```python
from build123d import *

# Parameters (mm, degrees)
SKETCH_1_R      = 35
SKETCH_1_R_2    = 15
SKETCH_1_R_3    = 1.6
EXTRUDE_1_DEPTH = 2
SKETCH_2_R      = 24
SKETCH_2_R_2    = 18.6
EXTRUDE_2_DEPTH = 7


with BuildPart() as part:
    # 草图1 → 凸台-拉伸1 (new body)
    with BuildSketch(Plane(origin=(0, 0, 0), x_dir=(1, 0, 0), z_dir=(0, 1, 0))):
        with Locations(Location((0, 0, 0), (0, 0, 270))):
            Circle(SKETCH_1_R)
        with Locations(Location((0, 0, 0), (0, 0, 270))):
            Circle(SKETCH_1_R_2, mode=Mode.SUBTRACT)
        with Locations(Location((29, 0, 0), (0, 0, 270))):
            Circle(SKETCH_1_R_3, mode=Mode.SUBTRACT)
        with Locations(Location((20.506096654, -20.506096654, 0), (0, 0, 270))):
            Circle(SKETCH_1_R_3, mode=Mode.SUBTRACT)
        with Locations(Location((0, -29, 0), (0, 0, 270))):
            Circle(SKETCH_1_R_3, mode=Mode.SUBTRACT)
        with Locations(Location((-20.506096654, -20.506096654, 0), (0, 0, 270))):
            Circle(SKETCH_1_R_3, mode=Mode.SUBTRACT)
        with Locations(Location((-29, 0, 0), (0, 0, 270))):
            Circle(SKETCH_1_R_3, mode=Mode.SUBTRACT)
        with Locations(Location((-20.506096654, 20.506096654, 0), (0, 0, 270))):
            Circle(SKETCH_1_R_3, mode=Mode.SUBTRACT)
        with Locations(Location((0, 29, 0), (0, 0, 270))):
            Circle(SKETCH_1_R_3, mode=Mode.SUBTRACT)
        with Locations(Location((20.506096654, 20.506096654, 0), (0, 0, 270))):
            Circle(SKETCH_1_R_3, mode=Mode.SUBTRACT)
    extrude(amount=-EXTRUDE_1_DEPTH)

    # 草图2 → 凸台-拉伸2 (add)
    with BuildSketch(Plane(origin=(0, 0, 0), x_dir=(1, 0, 0), z_dir=(0, 1, 0))):
        with Locations(Location((0, 0, 0), (0, 0, 270))):
            Circle(SKETCH_2_R)
        with Locations(Location((0, 0, 0), (0, 0, 270))):
            Circle(SKETCH_2_R_2, mode=Mode.SUBTRACT)
    extrude(amount=EXTRUDE_2_DEPTH)


solid = part.part
```
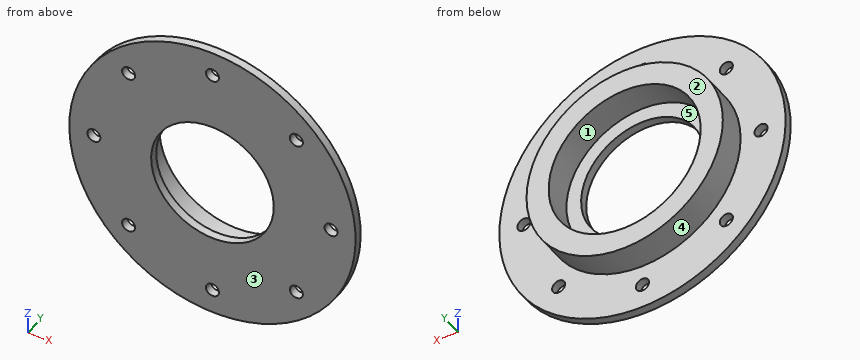
Work out the finished part from the listing and answer in its coordinate system (mm). Face numbers are marked on the shaded views. A direction names the side the tool comes from. Give positions to 0.01 mm unless a question says otherwise; leave off trailing zeros. Order: outer loops, then holes, each group sorted by start corner. A loop starts at its lowest first (then second) coordinate and runs counter-clockwise, first axis right, second up. Notation, with made-up numbers: (-6.75, 51.25) - (31.25, 51.25) arc R32 ccw to (31.25, 83.25) - close; hole circle Ø10 at (29, -5.5). An arc over 180 degrees is marked (long way). One line per item, written item: value. Start each with the question number.
1. Section B-B, the plane z = 29 is taken. Write down the section's boundary in (x, y), then the cut area to 3 significant figures.
2. Section A-A, the plane x = 0 is taken. Write down the section's boundary in (y, z), then the cut area to 3 significant figures.
3. For a pull along Z with two mould halves and no side action, classify the marked faces 3, 4 and 5 as released by +Z, released by -Z, zero draft, split by the parting line, or undercut.
4. Section C-C, the plane x = 10 is taken. Write down the section's boundary in (y, z).
5. Each of these flat-tipped pins is pushed along its axis until it touches: pin 1 Ø3 at (y, z) = (3.5, -4) entering from +X; pin 2 Ø5 at (x, z) = (-20.51, -20.51) entering from +Y. Where does it stop, or does it pass through?
6. Which of the six approach directions +Z, -Z, +X, -X, +Y, -Y give full straight-line access (tool end or side, diameter ignored) to the marked faces 1 and 2?
7. Section D-D, the plane z = -6 is taken. Write down the section's boundary in (x, y), then the cut area to 3 significant figures.
8. Consider line 1 (Y direction, x = 15, z = 3); line 2 (Z direction, x = 13, y = 0.25); line 3 (Z direction, x = 16.5, y = 4). Determine where each line is inside the solid, lowest interval first.
Filled sheet:
1. outline: (-19.6, -2) - (-1.6, -2) - (-1.6, 0) - (-19.6, 0) - close; (1.6, -2) - (19.6, -2) - (19.6, 0) - (1.6, 0) - close
1. area: 72.0 mm²
2. outline: (-2, -35) - (0, -35) - (0, -30.6) - (-2, -30.6) - close; (-2, -27.4) - (0, -27.4) - (0, -24) - (7, -24) - (7, -18.6) - (0, -18.6) - (0, -15) - (-2, -15) - close; (-2, 15) - (0, 15) - (0, 18.6) - (7, 18.6) - (7, 24) - (0, 24) - (0, 27.4) - (-2, 27.4) - close; (-2, 30.6) - (0, 30.6) - (0, 35) - (-2, 35) - close
2. area: 143 mm²
3. face 3: zero draft
3. face 4: split by the parting line
3. face 5: undercut
4. outline: (-2, -33.54) - (0, -33.54) - (0, -21.82) - (7, -21.82) - (7, -15.68) - (0, -15.68) - (0, -11.18) - (-2, -11.18) - close; (-2, 11.18) - (0, 11.18) - (0, 15.68) - (7, 15.68) - (7, 21.82) - (0, 21.82) - (0, 33.54) - (-2, 33.54) - close
5. pin 1: x = 23.87
5. pin 2: y = 0
6. face 1: +Y
6. face 2: +Z, -Z, +X, -X, +Y
7. outline: (-34.48, -2) - (-13.75, -2) - (-13.75, 0) - (-17.61, 0) - (-17.61, 7) - (-23.24, 7) - (-23.24, 0) - (-34.48, 0) - close; (13.75, -2) - (34.48, -2) - (34.48, 0) - (23.24, 0) - (23.24, 7) - (17.61, 7) - (17.61, 0) - (13.75, 0) - close
7. area: 162 mm²
8. line 1: -2 to 0
8. line 2: -20.17 to -13.3, 13.3 to 20.17
8. line 3: -17.43 to -8.59, 8.59 to 17.43
